from build123d import *

# Parameters (mm, degrees)
EXTRUDE_1_DEPTH = 5.5
EXTRUDE_2_DEPTH = 24.5
FILLET_1_SIZE   = 25
FILLET_1_SIZE_2 = 40
EXTRUDE_3_DEPTH = 15.5
SKETCH_2_3_R    = 2.750000000000008
SKETCH_2_3_R_2  = 2.7499999999999982
SKETCH_2_3_R_3  = 2.7499999999999987
SKETCH_2_3_R_4  = 2.7500000000000084
EXTRUDE_4_DEPTH = 21


with BuildPart() as part:
    # 草图1 → 凸台-拉伸1 (new body)
    with BuildSketch(Plane.XY):
        with BuildLine():
            Line((-10.000000000000071, 0), (-96.8, 0))
            Line((-96.8, 0), (-96.8, 70.29999999999998))
            Line((-96.8, 70.29999999999998), (-10.000000000000071, 70.3))
            ThreePointArc((-10.000000000000071, 70.3), (-2.928932188134527, 67.37106781186547), (0, 60.29999999999993))
            Line((0, 60.29999999999993), (0, 10.000000000000071))
            ThreePointArc((0, 10.000000000000071), (-2.9289321881345236, 2.9289321881345245), (-10.000000000000071, 0))
        make_face()
    extrude(amount=-EXTRUDE_1_DEPTH)

    # 草图1<4> → 凸台-拉伸2 (add)
    with BuildSketch(Plane.XY):
        with BuildLine():
            ThreePointArc((-35.15, 70.29999999999998), (-70.3, 35.15), (-35.150000000000006, -7.11e-15))
            Line((-35.15, 0), (-35.15, 70.3))
        make_face()
        with BuildLine():
            Line((-35.15, 70.3), (-35.15, 0))
            ThreePointArc((-35.150000000000006, -7.11e-15), (-10.295196641292861, 10.29519664129284), (0, 35.149999999999984))
            ThreePointArc((0, 35.14999999999999), (-10.295196641292854, 60.004803358707136), (-35.15, 70.29999999999998))
        make_face()
    extrude(amount=EXTRUDE_2_DEPTH)

    # 圆角1
    # a fillet whose section is not a circle: 40, 25 mm, written as the material it takes off along each edge
    with BuildSketch(Plane(origin=(-96.8, 70.29999999999998, 100.00000000000001), x_dir=(0, -1, 0), z_dir=(0, 0, -1))) as fillet_1_piece_1:
        with BuildLine():
            Bezier((FILLET_1_SIZE, 0), (0, 0), (0, -FILLET_1_SIZE_2), weights=[1, 0.7071067811865476, 1])
            Line((0, -FILLET_1_SIZE_2), (0, 0))
            Line((0, 0), (FILLET_1_SIZE, 0))
        make_face()
    extrude(amount=205.50000000000003, mode=Mode.SUBTRACT)
    with BuildSketch(Plane(origin=(-96.8, 0, 100.00000000000001), x_dir=(1, 0, 0), z_dir=(0, 0, -1))) as fillet_1_piece_2:
        with BuildLine():
            Bezier((FILLET_1_SIZE_2, 0), (0, 0), (0, -FILLET_1_SIZE), weights=[1, 0.7071067811865476, 1])
            Line((0, -FILLET_1_SIZE), (0, 0))
            Line((0, 0), (FILLET_1_SIZE_2, 0))
        make_face()
    extrude(amount=205.50000000000003, mode=Mode.SUBTRACT)

    # 圆角2: read off the stored shape, not the designer's step
    # 圆角2 outline → 圆角2 (revolve, cut)
    with BuildSketch(Plane(origin=(-35.15, 35.15, 0), x_dir=(1, 0, 0), z_dir=(0, -1, 0))):
        with BuildLine():
            ThreePointArc((34.15, 24.5), (34.857106781, 24.207106781), (35.15, 23.5))
            Line((35.15, 23.5), (35.15, 24.5))
            Line((35.15, 24.5), (34.15, 24.5))
        make_face()
    revolve(axis=Axis((-35.15, 35.15, 0), (0, 0, 1)), mode=Mode.SUBTRACT)

    # 草图2 → 凸台-拉伸3 (add)
    with BuildSketch(Plane(origin=(0, 0, -5.5), x_dir=(-1, 0, 0), z_dir=(0, 0, -1))):
        with BuildLine():
            ThreePointArc((65, 35.14999999999999), (80.9, 19.249999999999993), (96.80000000000001, 35.149999999999984))
            Line((96.8, 35.15), (65, 35.149999999999984))
        make_face()
        with BuildLine():
            Line((65, 35.149999999999984), (96.8, 35.15))
            ThreePointArc((96.80000000000001, 35.14999999999999), (80.9, 51.04999999999999), (65, 35.14999999999999))
        make_face()
    extrude(amount=EXTRUDE_3_DEPTH)

    # 草图2<3> → 凸台-拉伸4 (add)
    with BuildSketch(Plane(origin=(0, 0, -5.5), x_dir=(-1, 0, 0), z_dir=(0, 0, -1))):
        with Locations(Location((79.45, 15.149999999999999, 0), (0, 0, 180))):
            Circle(SKETCH_2_3_R)
        with Locations(Location((7.250000000000006, 7.64999999999999, 0), (0, 0, 180))):
            Circle(SKETCH_2_3_R_2)
        with Locations(Location((7.249999999999993, 62.65, 0), (0, 0, 180))):
            Circle(SKETCH_2_3_R_3)
        with Locations(Location((79.44999999999999, 55.15, 0), (0, 0, 180))):
            Circle(SKETCH_2_3_R_4)
    extrude(amount=EXTRUDE_4_DEPTH)


solid = part.part
Verification items for the finished model (mm, model axes). A direction names the side the tool comes from. Coordinates: 2 decimals unless noted, no trailing zeros. Order: outer loops, then holes, each group sorted by start corner. A loop starts at its lowest first (then second) coordinate and runs counter-clockwise, first axis right, second up. Notation, with made-up numbers: M -39.75,81 L -8.75,81 A11 cw -8.75,85 Z; hole C 78.25,-12.5 d3. An arc over 180 degrees is marked long. One line per item, written item: value. Start each with the question number.
Item 1: Gauge pin test, flat ends, axial feed: pin 1 (4 mm diameter, centred on y = 48.5, z = -15, fed in from -X); pin 2 (2 mm diameter, centred on x = -50, z = 10, fed in from +Y); pin 3 (1 mm diameter, centred on x = -84, z = -19, fed in from +Y); pin 4 (5 mm diameter, centred on x = -40, z = -8.5, fed in from -Y). Record the tip position at first contact, or that the pin passes through.
Item 2: Sectioned sample at A-A (z = 21). Enter the section's corners in (x, y).
Item 3: Scan lines: probe 1 along Z at (x, y) = (-19, 18.5); probe 2 along Z at (x, y) = (-74, 40.5); probe 3 along X at (y, z) = (8, -16.5). Record each from-to range of solid material in increasing order.
Item 4: Access from +Z, -Z, +X, -X, +Y, -Y to the whole of each face (thin tool, end or side, straight path). Record for faces 1 (the flat face through (-81, 35, -21)), 2 (the flat face through (-8, 7, 0)), 3 (the cylindrical face through (-2.85, 3.01, -2.71)), 4 (the cylindrical face through (-76.91, 16.2, -15.85)).
Conclusion:
1. pin 1: stops at x = -92.03
1. pin 2: stops at y = 67.46
1. pin 3: stops at y = 50.84
1. pin 4: passes through
2. outline: C -35.15,35.15 d70.3
3. probe 1: z = -5.5 to 24.5
3. probe 2: z = -21 to 0
3. probe 3: x = -9.98 to -4.52
4. face 1: -Z, +X, -X
4. face 2: +Z, +X, -Y
4. face 3: +Z, -Z, +X, -Y
4. face 4: -Z
